CAD build for the part. Positions are in the model's coordinates, mm. A direction names the side the tool comes from. Coordinates: 2 decimals unless noted, no trailing zeros. Write each loop counter-clockwise with the first axis right and the second up, starting at its lowest first coordinate (ties: lowest second). Pieces come first, ordered by that corner, then holes. Notation, with made-up numbers: (-24.5, 19) -> (-14.5, 19) arc R22 cw to (-14.5, 53) -> close; hole circle Ø9 at (83.5, -39.75). An arc over 180 degrees is marked (long way). Answer as CSV lines item,"result".
```python
from build123d import *

# Parameters (mm, degrees)
ESBO_O1_W                = 100
ESBO_O1_H                = 100
RESSALTO_EXTRUS_O1_DEPTH = 100
CHANFRO1_START           = -50
CHANFRO1_DEPTH           = 100
CHANFRO1_START_2         = -51
CHANFRO1_2_DEPTH         = 102
ESBO_O3_W                = 70
ESBO_O3_H                = 25
CORTE_EXTRUS_O1_DEPTH    = 123.474487139
ESBO_O4_W                = 70
ESBO_O4_H                = 20
CORTE_EXTRUS_O2_DEPTH    = 90
ESBO_O8_R                = 8.75
CORTE_EXTRUS_O6_DEPTH    = 141.445719052


with BuildPart() as part:
    # Esboço1 → Ressalto-extrusão1 (new body)
    with BuildSketch(Plane(origin=(0, 0, 0), x_dir=(1, 0, 0), z_dir=(0, 1, 0))):
        Rectangle(ESBO_O1_W, ESBO_O1_H)
    extrude(amount=RESSALTO_EXTRUS_O1_DEPTH)

    # Chanfro1: read off the stored shape, not the designer's step
    # Chanfro1 outline → Chanfro1 (cut)
    with BuildSketch(Plane.XY.offset(CHANFRO1_START)):
        Polygon((-50, 0), (-40, 100), (-50, 100), align=None)
        Polygon((40, 100), (50, 0), (50, 100), align=None)
    extrude(amount=CHANFRO1_DEPTH, mode=Mode.SUBTRACT)

    # Chanfro1 2 outline → Chanfro1 2 (cut)
    with BuildSketch(Plane.YZ.offset(CHANFRO1_START_2)):
        Polygon((0, 50), (100, 40), (100, 50), align=None)
        Polygon((100, -40), (0, -50), (100, -50), align=None)
    extrude(amount=CHANFRO1_2_DEPTH, mode=Mode.SUBTRACT)

    # Esboço3 → Corte-extrusão1 (cut, through all)
    with BuildSketch(Plane(origin=(0, 100, 0), x_dir=(1, 0, 0), z_dir=(0, 1, 0))):
        with Locations((0, 22.5)):
            Rectangle(ESBO_O3_W, ESBO_O3_H)
        with Locations((0, -22.5)):
            Rectangle(ESBO_O3_W, ESBO_O3_H)
    extrude(amount=-CORTE_EXTRUS_O1_DEPTH, mode=Mode.SUBTRACT)

    # Esboço4 → Corte-extrusão2 (cut)
    with BuildSketch(Plane(origin=(0, 100, 0), x_dir=(1, 0, 0), z_dir=(0, 1, 0))):
        Rectangle(ESBO_O4_W, ESBO_O4_H)
    extrude(amount=-CORTE_EXTRUS_O2_DEPTH, mode=Mode.SUBTRACT)

    # Esboço8 → Corte-extrusão6 (cut, through all)
    with BuildSketch(Plane.ZY.offset(-35)):
        with Locations((12.5, 64.5)):
            Circle(ESBO_O8_R)
        with Locations((-12.5, 64.5)):
            Circle(ESBO_O8_R)
    extrude(amount=-CORTE_EXTRUS_O6_DEPTH, mode=Mode.SUBTRACT)


solid = part.part
```
Item 1: Saw through at B-B on x = -29. Give the cut face in (y, z), and give its area (3 significant figures).
Answer below:
outline,"(0, -50) -> (100, -40) -> (100, -35) -> (0, -35) -> close; (0, -10) -> (10, -10) -> (10, 10) -> (0, 10) -> close; (0, 35) -> (100, 35) -> (100, 40) -> (0, 50) -> close"
area,"2,200 mm2"
Item 2: Flat gauge pins, fed straight in: pin 1 (1.5 mm diameter, centred on y = 28, z = 11.5, fed in from -X) (3 decimals); pin 2 (10 mm diameter, centred on x = -30, y = 79, fed in from -Z); pin 3 (6 mm diameter, centred on x = 9, z = 0.5, fed in from +Y); pin 4 (4 mm diameter, centred on x = -28.5, z = 31.5, fed in from +Y). Where does each tip first touch, or does it go through?
Answer below:
pin 1,"stops at x = -47.275"
pin 2,"stops at z = -42.6"
pin 3,"stops at y = 10"
pin 4,"passes through"
Item 3: Wall check: line 1 (Y direction, x = 38, z = 12.5); line 2 (Z direction, x = 40.25, y = 64.5); line 3 (X direction, y = 55, z = 20). Give the ranges that are in metal, low to high. Write a range as from..to.
Answer below:
line 1,"y = 0..55.75, 73.25..100"
line 2,"z = -43.55..-21.25, -3.75..3.75, 21.25..43.55"
line 3,"x = -44.5..-35, 35..44.5"
Item 4: 3-axis set-ups, long thin cutter, end or side, ignore diameter. For faces 1 (the cylindrical face through (39.65, 56.74, 16.54)), 2 (the flat face through (0, 10, 0)), 3 (the flat face through (0, 51, 35)), 4 (the flat face through (44.93, 50.7, -0.7)): which of +Z, -Z, +X, -X, +Y, -Y reach the whole face in a straight line?
Answer below:
face 1,"+X"
face 2,"+Y"
face 3,"+Y, -Y"
face 4,"+Z, -Z, +X, +Y"
Item 5: Saw through at D-D on z = -13. Give the cut face in (x, y).
Answer below:
outline,"(-50, 0) -> (-35, 0) -> (-35, 100) -> (-40, 100) -> close; (35, 0) -> (50, 0) -> (44.42, 55.76) -> (35, 55.76) -> close; (35, 73.24) -> (42.68, 73.24) -> (40, 100) -> (35, 100) -> close"
Item 6: Two-plate mould, pull along Z, no slides. Class faces 5 (the flat face through (-35, 51, 0)), 6 (the flat face through (-0.7, 49.3, 45.07)), 7 (the flat face through (-1, 0, -1)), 8 (the flat face through (35, 51, 0)): pulls with the +Z half, pulls with the -Z half, needs draft (parallel to the pull), parting line crosses it, or undercut.
Answer below:
face 5,"undercut"
face 6,"pulls with the +Z half"
face 7,"needs draft"
face 8,"undercut"
Item 7: Saw through at C-C on y = 90. Give the cut face in (x, z), and give its area (3 significant figures).
Answer below:
outline,"(-41, -41) -> (41, -41) -> (41, 41) -> (-41, 41) -> close; hole (-35, -35) -> (35, -35) -> (35, 35) -> (-35, 35) -> close"
area,"1,820 mm2"
Item 8: Saw through at A-A on y = 64.5. Give the cut face in (x, z), and give its area (3 significant figures).
Answer below:
outline,"(-43.55, -43.55) -> (43.55, -43.55) -> (43.55, -21.25) -> (35, -21.25) -> (35, -35) -> (-35, -35) -> (-35, 35) -> (35, 35) -> (35, 21.25) -> (43.55, 21.25) -> (43.55, 43.55) -> (-43.55, 43.55) -> close; (35, -3.75) -> (43.55, -3.75) -> (43.55, 3.75) -> (35, 3.75) -> close"
area,"2,390 mm2"
